Part model, mm, in its own coordinate system. A direction names the side the tool comes from. Coordinates: 2 decimals unless noted, no trailing zeros. Write each question's results on one line, items separated by ' | '.
from build123d import *

# Parameters (mm, degrees)
F1_R = 15


with BuildPart() as f3:
    # F3: sweep along a path in F0
    with BuildLine(Plane.YZ) as f3_path:
        Line((0, 0), (60, 0))
        ThreePointArc((60, 0), (77.320508, 3.944487), (91.22499, 15))
        ThreePointArc((91.22499, 15), (109.739598, 27.926853), (132.304801, 28.767029))
        ThreePointArc((132.304801, 28.767029), (206.720078, 14.709975), (282.304801, 10))
        Line((282.304801, 10), (650, 10))
    # F1 (on Front) → F3 (sweep)
    with BuildSketch(Plane.XZ):
        Circle(F1_R)
    sweep(path=f3_path.line)


solid = f3.part
(1) Wall check: line 1 (Z direction, x = 0, y = 466.5); line 2 (X direction, y = 501.5, z = 9.5); line 3 (X direction, y = 505, z = 8). Give the ranges that are in metal, low to high. Write a range as from..to.
Return value:
line 1: z = -5..25 | line 2: x = -14.99..14.99 | line 3: x = -14.87..14.87
(2) Flat gauge pins, fed straight in: P1, Ø4, axis at x = -4, y = 383.5, coming from the -Z side; P2, Ø4, axis at x = -6, y = 239.5, coming from the +Z side; P3, Ø4, axis at x = -7, z = 32.5, coming from the -Y side. Where does each tip first touch, or does it go through?
Return value:
P1: stops at z = -4.87 | P2: stops at z = 26.02 | P3: stops at y = 87.42
(3) 3-axis set-ups, long thin cutter, end or side, ignore diameter. For faces 1 (the cylindrical face through (-14.985, 30.42, -0.66)), 2 (the flat face through (0, 650, 10)): which of +Z, -Z, +X, -X, +Y, -Y reach the whole face in a straight line?
Return value:
face 1: -Y | face 2: +Z, -Z, +X, -X, +Y
